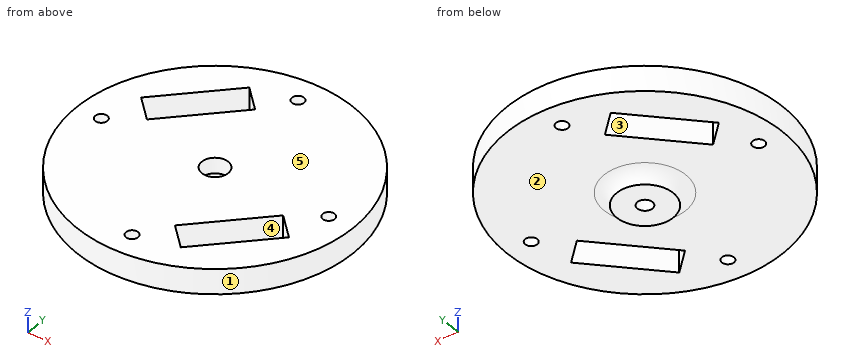
from build123d import *

# Parameters (mm, degrees)
SKETCH1_R                               = 7.5
BOSS_EXTRUDE1_DEPTH                     = 20.05
SKETCH3_W                               = 5
SKETCH3_H                               = 5
CUT_EXTRUDE1_DEPTH                      = 21
SKETCH6_R                               = 8.5
BOSS_EXTRUDE2_DEPTH                     = 24
SKETCH7_R                               = 11.25
BOSS_EXTRUDE3_DEPTH                     = 5
SKETCH8_R                               = 55
BOSS_EXTRUDE4_DEPTH                     = 10
FILLET1_R                               = 0.6
FILLET2_R                               = 5
M4_CLEARANCE_HOLE1_D                    = 4.8
M6X1_0_TAPPED_HOLE2_D                   = 5
M6X1_0_TAPPED_HOLE2_DEPTH               = 23.497848452
M6X1_0_TAPPED_HOLE2_TIP                 = 1.502151548
SKETCH13_R                              = 7.5
CUT_EXTRUDE2_DEPTH                      = 2
CUT_EXTRUDE3_REACH                      = 98.461
SKETCH15_R                              = 36.682415144
CUT_EXTRUDE4_DEPTH                      = 42.05
CBORE_FOR_M6_HEX_HEAD_BOLT1_D           = 6
CBORE_FOR_M6_HEX_HEAD_BOLT1_CBORE_D     = 10.5
CBORE_FOR_M6_HEX_HEAD_BOLT1_CBORE_DEPTH = 6.2


with BuildPart() as part:
    # Sketch1 → Boss-Extrude1 (new body)
    with BuildSketch(Plane.XY):
        Circle(SKETCH1_R)
    extrude(amount=BOSS_EXTRUDE1_DEPTH)

    # Sketch3 → Cut-Extrude1 (cut)
    with BuildSketch(Plane(origin=(0, 0, 0), x_dir=(-1, 0, 0), z_dir=(0, 0, -1))):
        with Locations((0, 7.5)):
            Rectangle(SKETCH3_W, SKETCH3_H)
    extrude(amount=-CUT_EXTRUDE1_DEPTH, mode=Mode.SUBTRACT)

    # Sketch6 → Boss-Extrude2 (add)
    with BuildSketch(Plane.XY.offset(20.05)):
        Circle(SKETCH6_R)
    extrude(amount=BOSS_EXTRUDE2_DEPTH)

    # Sketch7 → Boss-Extrude3 (add)
    with BuildSketch(Plane.XY.offset(44.05)):
        Circle(SKETCH7_R)
    extrude(amount=BOSS_EXTRUDE3_DEPTH)

    # Sketch8 → Boss-Extrude4 (add)
    with BuildSketch(Plane.XY.offset(49.05)):
        Circle(SKETCH8_R)
    extrude(amount=BOSS_EXTRUDE4_DEPTH)

    # Fillet1
    fillet1_edges = [part.edges().sort_by_distance(p)[0] for p in [
        (-8.5, 0, 44.05),
    ]]
    fillet(fillet1_edges, radius=FILLET1_R)

    # Fillet2
    fillet2_edges = [part.edges().sort_by_distance(p)[0] for p in [
        (-11.25, 0, 49.05),
    ]]
    fillet(fillet2_edges, radius=FILLET2_R - 0.0001)  # a hair under: the kernel refuses the full size

    # M4 Clearance Hole1 (through all)
    with Locations(Plane.XY.offset(59.05)):
        with Locations((0, 45), (0, -45), (45, 0), (-45, 0)):
            Hole(M4_CLEARANCE_HOLE1_D / 2)

    # M6x1.0 Tapped Hole2
    with Locations(Plane(origin=(0, 0, 0), x_dir=(-1, 0, 0), z_dir=(0, 0, -1))):
        with Locations((0, 0)):
            Hole(M6X1_0_TAPPED_HOLE2_D / 2, depth=M6X1_0_TAPPED_HOLE2_DEPTH)
            with Locations((0, 0, -(M6X1_0_TAPPED_HOLE2_DEPTH + M6X1_0_TAPPED_HOLE2_TIP / 2))):  # 118° drill point
                Cone(0, M6X1_0_TAPPED_HOLE2_D / 2, M6X1_0_TAPPED_HOLE2_TIP, mode=Mode.SUBTRACT)

    # Sketch13 → Cut-Extrude2 (cut)
    with BuildSketch(Plane(origin=(0, 0, 0), x_dir=(-1, 0, 0), z_dir=(0, 0, -1))):
        Circle(SKETCH13_R)
    extrude(amount=-CUT_EXTRUDE2_DEPTH, mode=Mode.SUBTRACT)

    # Sketch14 → Cut-Extrude3 (cut, up to next)
    with BuildSketch(Plane.XY.offset(59.05), mode=Mode.PRIVATE) as cut_extrude3_sk1:
        Polygon((-16.617009358, 41.365746699), (-41.365746699, 16.617009358), (-32.880465325, 8.131727984), (-8.131727984, 32.880465325), align=None)
    cut_extrude3_tool1 = extrude(cut_extrude3_sk1.sketch, amount=-CUT_EXTRUDE3_REACH, mode=Mode.PRIVATE) & part.part
    # Sketch14 → Cut-Extrude3 (cut, up to next)
    with BuildSketch(Plane.XY.offset(59.05), mode=Mode.PRIVATE) as cut_extrude3_sk2:
        Polygon((41.365746699, -16.617009358), (16.617009358, -41.365746699), (8.131727984, -32.880465325), (32.880465325, -8.131727984), align=None)
    cut_extrude3_tool2 = extrude(cut_extrude3_sk2.sketch, amount=-CUT_EXTRUDE3_REACH, mode=Mode.PRIVATE) & part.part
    add(cut_extrude3_tool1.solids().sort_by_distance((-24.748737, 24.748737, 59.05))[0], mode=Mode.SUBTRACT)
    add(cut_extrude3_tool2.solids().sort_by_distance((24.748737, -24.748737, 59.05))[0], mode=Mode.SUBTRACT)

    # Sketch15 → Cut-Extrude4 (cut)
    with BuildSketch(Plane(origin=(0, 0, 2), x_dir=(-1, 0, 0), z_dir=(0, 0, -1))):
        Circle(SKETCH15_R)
    extrude(amount=-CUT_EXTRUDE4_DEPTH, mode=Mode.SUBTRACT)

    # CBORE for M6 Hex Head Bolt1 (through all)
    with Locations(Plane.XY.offset(59.05)):
        with Locations((0, 0)):
            CounterBoreHole(CBORE_FOR_M6_HEX_HEAD_BOLT1_D / 2, CBORE_FOR_M6_HEX_HEAD_BOLT1_CBORE_D / 2, CBORE_FOR_M6_HEX_HEAD_BOLT1_CBORE_DEPTH)


solid = part.part
Build history of the part. All positions in model axes, mm. Face numbers are marked on the shaded views. A direction names the side the tool comes from. Give positions to 0.01 mm unless a question says otherwise; leave off trailing zeros. Write each loop counter-clockwise with the first axis right and the second up, starting at its lowest first coordinate (ties: lowest second). Pieces come first, ordered by that corner, then holes. Notation, with made-up numbers: (72.25, 21.25) - (98.25, 21.25) arc R19 ccw to (98.25, 38.25) - close; hole circle Ø11 at (25, 3.25). An arc over 180 degrees is marked (long way). Use one line per item in the form item = value. Start each with the question number.
1. 3-axis set-ups, long thin cutter, end or side, ignore diameter. For the marked faces 4 and 5: which of +Z, -Z, +X, -X, +Y, -Y reach the whole face in a straight line?
2. Band-saw the part on A-A on y = 0. Count the separate pieces of the cut face and the enclosed holes in it, plus the area to 3 significant figures.
3. Probe line 1 (Y direction, x = 0, z = 50.25); line 2 (X direction, y = 1, z = 49.5); line 3 (X direction, y = 0.5, z = 57.25). List the from-to ranges inside material, lowest first. Write a range as [from, to].
4. Two-plate mould, pull along Y, no slides. Class the marked faces 1, 2 and 3: released by +Y, released by -Y, zero draft, split by the parting line, or undercut.
5. Drop flat-ended pins along their axis: pin 1 Ø3 at (x, z) = (-20.5, 55.5) entering from +Y; pin 2 Ø2 at (y, z) = (30, 48.5) entering from +X; pin 3 Ø1 at (y, z) = (28, 53) entering from -X. Give the stop position or say it passes through.
6. Band-saw the part on C-C on z = 55.75. Write the cut outline in (x, y).
7. Band-saw the part on D-D on x = 20.5. Write the cut outline in (y, z), plus the area to 3 significant figures.
Conclusion:
q1.face_4 = +Z, -Z
q1.face_5 = +Z, +X, -X, +Y, -Y
q2.separate_pieces = 4
q2.enclosed_holes = 0
q2.area = 1,010 mm²
q3.line_1 = [-55, -47.4], [-42.6, -3], [3, 42.6], [47.4, 55]
q3.line_2 = [-54.99, -47.18], [-42.82, -2.83], [2.83, 42.82], [47.18, 54.99]
q3.line_3 = [-55, -47.35], [-42.65, -5.23], [5.23, 42.65], [47.35, 55]
q4.face_1 = split by the parting line
q4.face_2 = zero draft
q4.face_3 = undercut
q5.pin_1 = 51.61
q5.pin_2 = 46.63
q5.pin_3 = -47.63
q6.outline = circle Ø110 at (0, 0); hole circle Ø4.8 at (-45, 0); hole (-41.37, 16.62) - (-32.88, 8.13) - (-8.13, 32.88) - (-16.62, 41.37) - close; hole circle Ø10.5 at (0, 0); hole circle Ø4.8 at (0, -45); hole circle Ø4.8 at (0, 45); hole (8.13, -32.88) - (16.62, -41.37) - (41.37, -16.62) - (32.88, -8.13) - close; hole circle Ø4.8 at (45, 0)
q7.outline = (-51.04, 49.05) - (-37.48, 49.05) - (-37.48, 59.05) - (-51.04, 59.05) - close; (-20.51, 49.05) - (51.04, 49.05) - (51.04, 59.05) - (-20.51, 59.05) - close
q7.area = 851 mm²
